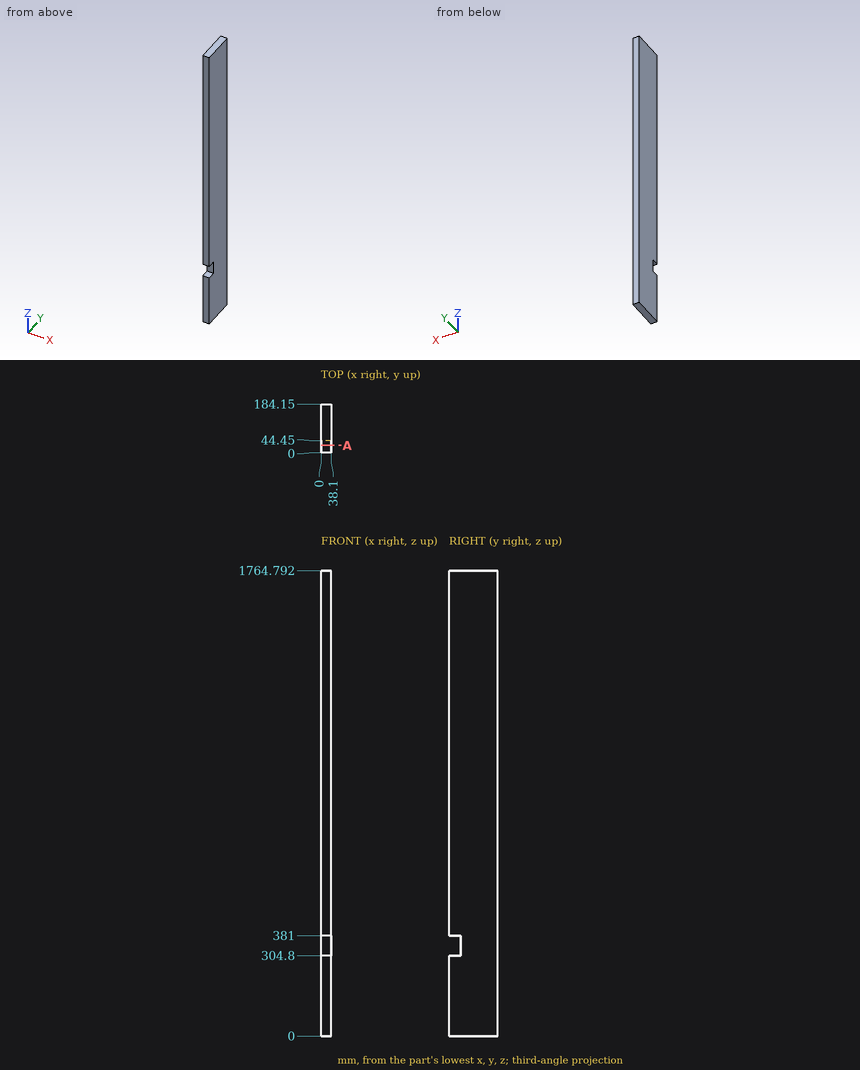
Answer from the drawing. Dimensions are ordinates in mm from the lowest x, y and z of the part. Give positions to 0.01 mm unless a question says otherwise; leave off trailing zeros. Write each loop counter-clockwise with the first axis right and the second up, starting at its lowest first coordinate (ties: lowest second). Pieces come first, ordered by that corner, then holes. Notation, with made-up numbers: (25.5, 44) -> (78.5, 44) arc R30 ccw to (78.5, 68) -> close; hole circle Ø6 at (-38, -33.75). An arc over 180 degrees is marked (long way). Use a Markdown table: item, result.
(1) Section A-A, the plane y = 27.5 is taken. Determine the outline of the cut face in (x, z).
Return value:
| item | result |
|---|---|
| outline | (0, 0) -> (38.1, 0) -> (38.1, 304.8) -> (0, 304.8) -> close; (0, 381) -> (38.1, 381) -> (38.1, 1764.79) -> (0, 1764.79) -> close |
(2) Find the intervals of material crossed by probe 1 along Z at (x, y) = (27, 34); probe 2 along Y at (x, z) = (10, 319), in increasing order. Write a range as from..to.
Return value:
| item | result |
|---|---|
| probe 1 | 0..304.8, 381..1764.79 |
| probe 2 | 44.45..184.15 |
(3) Flat-ended cylindrical pins translate along their axes: P1, Ø5, axis at y = 127.5, z = 1054, coming from the -X side; P2, Ø4, axis at x = 28, z = 357.5, coming from the -Y side. Find the tip coordinate at first contact, or state that the pin passes through.
Return value:
| item | result |
|---|---|
| P1 | x = 0 |
| P2 | y = 44.45 |
